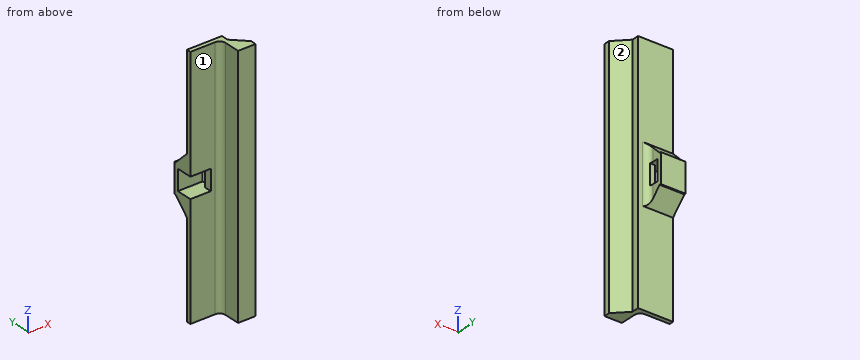
```python
from build123d import *

# Parameters (mm, degrees)
SKETCH_1_W          = 6
SKETCH_1_H          = 85
EXTRUDE_1_DEPTH     = 1.5
SKETCH_2_W          = 1.5
SKETCH_2_H          = 85
EXTRUDE_2_DEPTH     = 6
EXTRUDE_3_DEPTH     = 1.5
SKETCH_4_W          = 7
SKETCH_4_H          = 7
EXTRUDE_4_DEPTH     = 5.5
SKETCH_5_W          = 7
SKETCH_5_H          = 7
CUT_EXTRUDE_1_DEPTH = 4
SKETCH_6_W          = 7
SKETCH_6_H          = 3
CUT_EXTRUDE_2_DEPTH = 4
CHAMFER_1_SIZE      = 5
CHAMFER_2_SIZE      = 5
FILLET_1_R          = 2
FILLET_2_R          = 2


with BuildPart() as part:
    # Эскиз1 → Бобышка-Вытянуть1 (new body)
    with BuildSketch(Plane(origin=(0, 0, 0), x_dir=(1, 0, 0), z_dir=(0, 1, 0))):
        Rectangle(SKETCH_1_W, SKETCH_1_H)
    extrude(amount=EXTRUDE_1_DEPTH)

    # Эскиз2 → Бобышка-Вытянуть2 (add)
    with BuildSketch(Plane(origin=(0, 1.5, 0), x_dir=(1, 0, 0), z_dir=(0, 1, 0))):
        with Locations((-2.25, 0)):
            Rectangle(SKETCH_2_W, SKETCH_2_H)
    extrude(amount=EXTRUDE_2_DEPTH)

    # Эскиз3 → Бобышка-Вытянуть3 (add)
    with BuildSketch(Plane(origin=(0, 7.5, 0), x_dir=(1, 0, 0), z_dir=(0, 1, 0))):
        Polygon((-1.5, -42.5), (-13.5, -42.5), (-13.5, -3.5), (-6.5, -3.5), (-6.5, 3.5), (-13.5, 3.5), (-13.5, 42.5), (-1.5, 42.5), align=None)
    extrude(amount=EXTRUDE_3_DEPTH)

    # Эскиз4 → Бобышка-Вытянуть4 (add)
    with BuildSketch(Plane(origin=(0, 9, 0), x_dir=(1, 0, 0), z_dir=(0, 1, 0))):
        Polygon((-13.5, -3.5), (-13.5, -5), (-5, -5), (-5, 5), (-13.5, 5), (-13.5, 3.5), (-6.5, 3.5), (-6.5, -3.5), align=None)
        with Locations((-10, 0)):
            Rectangle(SKETCH_4_W, SKETCH_4_H)
    extrude(amount=EXTRUDE_4_DEPTH)

    # Эскиз5 → Вырез-Вытянуть1 (cut)
    with BuildSketch(Plane.XZ.offset(-9)):
        with Locations((-10, 0)):
            Rectangle(SKETCH_5_W, SKETCH_5_H)
    extrude(amount=-CUT_EXTRUDE_1_DEPTH, mode=Mode.SUBTRACT)

    # Эскиз6 → Вырез-Вытянуть2 (cut)
    with BuildSketch(Plane(origin=(-5, 0, 0), x_dir=(0, 0, -1), z_dir=(1, 0, 0))):
        with Locations((0, 11.5)):
            Rectangle(SKETCH_6_W, SKETCH_6_H)
    extrude(amount=-CUT_EXTRUDE_2_DEPTH, mode=Mode.SUBTRACT)

    # Фаска1
    # the kernel refuses this chamfer: 5 mm, written as the material it adds along each edge
    with BuildSketch(Plane(origin=(-1.5, 1.5, 42.5), x_dir=(-0.02749587661058636, 0.9996219169112968, 0), z_dir=(0, 0, -1))) as chamfer_1_piece_1_section:
        Polygon((CHAMFER_1_SIZE * 0.999621916911, CHAMFER_1_SIZE * 0.0274958766106), (-CHAMFER_1_SIZE * 0.0274958766106, CHAMFER_1_SIZE * 0.999621916911), (0, 0), align=None)
    chamfer_1_piece_1 = extrude(amount=85, mode=Mode.PRIVATE)
    chamfer_1_piece_1 = split(chamfer_1_piece_1, bisect_by=Plane(origin=(3, 3.179503735, 0), z_dir=(-1, 0, 0)), keep=Keep.TOP, mode=Mode.PRIVATE)
    add(chamfer_1_piece_1)

    # Фаска2
    chamfer_2_edges = [part.edges().sort_by_distance(p)[0] for p in [
        (-9.25, 9, 5),
        (-9.25, 9, -5),
    ]]
    chamfer(chamfer_2_edges, length=CHAMFER_2_SIZE)

    # Скругление1
    # the kernel refuses this fillet: 2 mm, written as the material it adds along each edge
    with BuildSketch(Plane(origin=(-5, 9, -15), x_dir=(1, 0, 0), z_dir=(0, 0, 1))) as fillet_1_piece_1_section:
        with BuildLine():
            CenterArc((FILLET_1_R, FILLET_1_R), FILLET_1_R, 180, 90)
            Line((0, FILLET_1_R), (0, 0))
            Line((0, 0), (FILLET_1_R, 0))
        make_face()
    fillet_1_piece_1 = extrude(amount=30, mode=Mode.PRIVATE)
    fillet_1_piece_1 = split(fillet_1_piece_1, bisect_by=Plane(origin=(-4.478955551, 10.861954239, -8.138045761), z_dir=(0, -0.7071067811865476, 0.7071067811865475)), keep=Keep.TOP, mode=Mode.PRIVATE)
    fillet_1_piece_1 = split(fillet_1_piece_1, bisect_by=Plane(origin=(-4.478955551, 10, -6.592030507), z_dir=(0, -1, 0)), keep=Keep.TOP, mode=Mode.PRIVATE)
    fillet_1_piece_1 = split(fillet_1_piece_1, bisect_by=Plane(origin=(-4.478955551, 9.315938986, -3.5), z_dir=(0, 0, -1)), keep=Keep.TOP, mode=Mode.PRIVATE)
    add(fillet_1_piece_1)
    with BuildSketch(Plane(origin=(-5, 9, -15), x_dir=(1, 0, 0), z_dir=(0, 0, 1))) as fillet_1_piece_2_section:
        with BuildLine():
            CenterArc((FILLET_1_R, FILLET_1_R), FILLET_1_R, 180, 90)
            Line((0, FILLET_1_R), (0, 0))
            Line((0, 0), (FILLET_1_R, 0))
        make_face()
    fillet_1_piece_2 = extrude(amount=30, mode=Mode.PRIVATE)
    fillet_1_piece_2 = split(fillet_1_piece_2, bisect_by=Plane(origin=(-4.950049331, 11.610374757, -7.389625243), z_dir=(0, -0.7071067811865476, 0.7071067811865475)), keep=Keep.TOP, mode=Mode.PRIVATE)
    fillet_1_piece_2 = split(fillet_1_piece_2, bisect_by=Plane(origin=(-4.950049331, 10, -6.093083495), z_dir=(0, 1, 0)), keep=Keep.TOP, mode=Mode.PRIVATE)
    fillet_1_piece_2 = split(fillet_1_piece_2, bisect_by=Plane(origin=(-4.950049331, 10.313833009, -3.5), z_dir=(0, 0, -1)), keep=Keep.TOP, mode=Mode.PRIVATE)
    add(fillet_1_piece_2)
    with BuildSketch(Plane(origin=(-5, 9, -15), x_dir=(1, 0, 0), z_dir=(0, 0, 1))) as fillet_1_piece_3_section:
        with BuildLine():
            CenterArc((FILLET_1_R, FILLET_1_R), FILLET_1_R, 180, 90)
            Line((0, FILLET_1_R), (0, 0))
            Line((0, 0), (FILLET_1_R, 0))
        make_face()
    fillet_1_piece_3 = extrude(amount=30, mode=Mode.PRIVATE)
    fillet_1_piece_3 = split(fillet_1_piece_3, bisect_by=Plane(origin=(-4.48975988, 9.328783529, 3.5), z_dir=(0, 0, -1)), keep=Keep.TOP, mode=Mode.PRIVATE)
    fillet_1_piece_3 = split(fillet_1_piece_3, bisect_by=Plane(origin=(-4.48975988, 10, 0), z_dir=(0, -1, 0)), keep=Keep.TOP, mode=Mode.PRIVATE)
    fillet_1_piece_3 = split(fillet_1_piece_3, bisect_by=Plane(origin=(-4.48975988, 9.328783529, -3.5), z_dir=(0, 0, 1)), keep=Keep.TOP, mode=Mode.PRIVATE)
    add(fillet_1_piece_3)
    with BuildSketch(Plane(origin=(-5, 9, -15), x_dir=(1, 0, 0), z_dir=(0, 0, 1))) as fillet_1_piece_4_section:
        with BuildLine():
            CenterArc((FILLET_1_R, FILLET_1_R), FILLET_1_R, 180, 90)
            Line((0, FILLET_1_R), (0, 0))
            Line((0, 0), (FILLET_1_R, 0))
        make_face()
    fillet_1_piece_4 = extrude(amount=30, mode=Mode.PRIVATE)
    fillet_1_piece_4 = split(fillet_1_piece_4, bisect_by=Plane(origin=(-4.478955551, 10.861954239, 8.138045761), z_dir=(0, -0.7071067811865475, -0.7071067811865476)), keep=Keep.TOP, mode=Mode.PRIVATE)
    fillet_1_piece_4 = split(fillet_1_piece_4, bisect_by=Plane(origin=(-4.478955551, 9.315938986, 3.5), z_dir=(0, 0, 1)), keep=Keep.TOP, mode=Mode.PRIVATE)
    fillet_1_piece_4 = split(fillet_1_piece_4, bisect_by=Plane(origin=(-4.478955551, 10, 6.592030507), z_dir=(0, -1, 0)), keep=Keep.TOP, mode=Mode.PRIVATE)
    add(fillet_1_piece_4)
    with BuildSketch(Plane(origin=(-5, 9, -15), x_dir=(1, 0, 0), z_dir=(0, 0, 1))) as fillet_1_piece_5_section:
        with BuildLine():
            CenterArc((FILLET_1_R, FILLET_1_R), FILLET_1_R, 180, 90)
            Line((0, FILLET_1_R), (0, 0))
            Line((0, 0), (FILLET_1_R, 0))
        make_face()
    fillet_1_piece_5 = extrude(amount=30, mode=Mode.PRIVATE)
    fillet_1_piece_5 = split(fillet_1_piece_5, bisect_by=Plane(origin=(-4.950049331, 11.610374757, 7.389625243), z_dir=(0, -0.7071067811865475, -0.7071067811865476)), keep=Keep.TOP, mode=Mode.PRIVATE)
    fillet_1_piece_5 = split(fillet_1_piece_5, bisect_by=Plane(origin=(-4.950049331, 10.313833009, 3.5), z_dir=(0, 0, 1)), keep=Keep.TOP, mode=Mode.PRIVATE)
    fillet_1_piece_5 = split(fillet_1_piece_5, bisect_by=Plane(origin=(-4.950049331, 10, 6.093083495), z_dir=(0, 1, 0)), keep=Keep.TOP, mode=Mode.PRIVATE)
    add(fillet_1_piece_5)

    # Скругление2
    fillet_2_edges = [part.edges().sort_by_distance(p)[0] for p in [
        (-3, 7.5, 0),
    ]]
    fillet(fillet_2_edges, radius=FILLET_2_R)


solid = part.part
```
Geometry: final body of the model. Coordinates: model frame, mm. Face numbers are marked on the shaded views. A direction names the side the tool comes from. Give positions to 0.01 mm unless a question says otherwise; leave off trailing zeros. Order: outer loops, then holes, each group sorted by start corner. A loop starts at its lowest first (then second) coordinate and runs counter-clockwise, first axis right, second up. Notation, with made-up numbers: M -29.75,-31.75 L 0.25,-31.75 A16 ccw 0.25,-25.75 Z; hole C -36,30 d5. An arc over 180 degrees is marked long. Answer as CSV lines item,"result". Start each with the question number.
1) Set-up query: the marked faces 1 and 2. Return all of +Z, -Z, +X, -X, +Y, -Y with unobstructed straight access to the full face (end or side cutting, diameter ignored); none if empty.
2) Cut plane B-B (x = -8). Output: boundary loops of the cut face in (y, z), then the cut area to 3 significant figures.
3) Line query: line 1 (Y direction, x = -5.75, z = 0); line 2 (Z direction, x = -8.75, y = 7.75); line 3 (Y direction, x = -7.5, z = -28.5). Output: solid intervals per line, ascending. Write a range as from..to.
4) First-contact query: P1, Ø2.5, axis at x = -10, z = 15.5, coming from the -Y side; P2, Ø0.8, axis at y = 9, z = 0, coming from the -X side; P3, Ø3, axis at x = -8, y = 11.5, coming from the +Z side. Flat tips, straight axial feed; report the tip coordinate or a pass-through.
5) Cut plane D-D (y = 4.25). Output: boundary loops of the cut face in (x, z).
6) Cut plane C-C (z = 17). Output: boundary loops of the cut face in (x, y).
7) Cut plane A-A (y = 11.75). Output: boundary loops of the cut face in (x, z), then the cut area to 4 significant figures.
Findings below:
1,face 1,"+Z, -Z, -X, -Y"
1,face 2,"+Z, -Z, +X, +Y"
2,outline,"M 7.5,-42.5 L 9,-42.5 L 9,-10 L 14,-5 L 14.5,-5 L 14.5,5 L 14,5 L 9,10 L 9,42.5 L 7.5,42.5 L 7.5,3.5 L 13,3.5 L 13,-3.5 L 7.5,-3.5 Z"
2,area,"169 mm²"
3,line 1,"y = 7.5..10, 13..14.5"
3,line 2,"z = -42.5..-3.5, 3.5..42.5"
3,line 3,"y = 7.5..9"
4,P1,"stops at y = 7.5"
4,P2,"stops at x = -6.5"
4,P3,"stops at z = 9"
5,outline,"M -3,-42.5 L 0.75,-42.5 L 0.75,42.5 L -3,42.5 Z"
6,outline,"M -13.5,7.5 L -5,7.5 A2 cw -3,5.5 L -3,0 L 3,0 L 3,2 L -1.5,6.5 L -1.5,9 L -13.5,9 Z"
7,outline,"M -13.5,-7.25 L -5,-7.25 L -5,-3.5 L -13.5,-3.5 Z; M -13.5,3.5 L -5,3.5 L -5,7.25 L -13.5,7.25 Z"
7,area,"63.75 mm²"
